The model under review builds one solid part; all positions refer to its coordinate system, in mm. Face numbers are marked on the shaded views. A direction names the side the tool comes from. Give positions to 0.01 mm unless a question says otherwise; leave off trailing zeros. Loops run counter-clockwise (first coordinate to the right, second up) from the corner with the lowest first, then second, coordinate; pieces in that order, holes last. Notation, with made-up numbers: (82.5, 39.25) - (121.5, 39.25) arc R22 cw to (121.5, 45.25) - close; hole circle Ø10 at (88, 36). An arc over 180 degrees is marked (long way). Return JSON: item names as keys, results as strings. Group by question number.
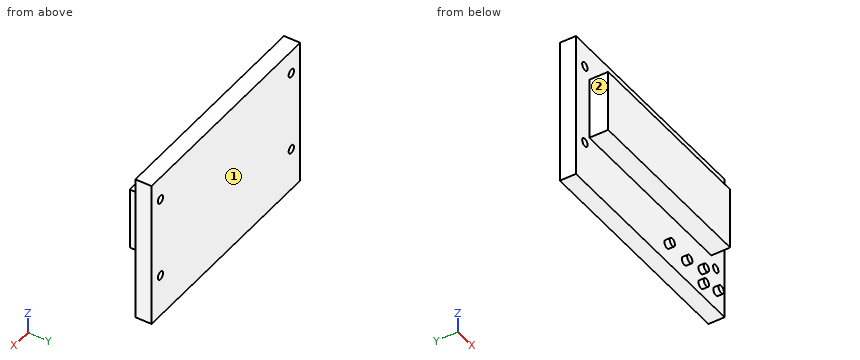
```python
from build123d import *

# Parameters (mm, degrees)
F0_W     = 85.09
F0_H     = 56.134
F0_R     = 1.524
F1_DEPTH = 6.096
F2_W     = 69.85
F2_H     = 23.622
F3_DEPTH = 7.112
F4_R     = 1.5
F5_DEPTH = 2


with BuildPart() as f1:
    # F0 (on Front) → F1 (new body)
    with BuildSketch(Plane.XZ):
        Rectangle(F0_W, F0_H)
        with Locations((-37.465, -11.811)):
            Circle(F0_R, mode=Mode.SUBTRACT)
        with Locations((37.465, -11.811)):
            Circle(F0_R, mode=Mode.SUBTRACT)
        with Locations((-37.465, 19.177)):
            Circle(F0_R, mode=Mode.SUBTRACT)
        with Locations((37.465, 19.177)):
            Circle(F0_R, mode=Mode.SUBTRACT)
    extrude(amount=F1_DEPTH)

    # F2 (on face) → F3 (join)
    with BuildSketch(Plane.XZ.offset(6.096)):
        with Locations((0, 3.683)):
            Rectangle(F2_W, F2_H)
    extrude(amount=F3_DEPTH)

    # F4 (on face) → F5 (join)
    with BuildSketch(Plane.XZ.offset(6.096)):
        with Locations((9.545, -21.067)):
            Circle(F4_R)
        with Locations((19.545, -21.067)):
            Circle(F4_R)
        with Locations((29.045, -24.067)):
            Circle(F4_R)
        with Locations((29.045, -18.067)):
            Circle(F4_R)
        with Locations((37.545, -21.067)):
            Circle(F4_R)
    extrude(amount=F5_DEPTH)


solid = f1.part
```
1) To check wall thickness, follow line 1 (Z direction, x = -38.5, y = -4.25); line 2 (X direction, y = -12, z = 6) (3 decimals); line 3 (Z direction, x = 31.5, y = -8.5). State the ranges of each line that lie inside material, in increasing order.
2) We need section A-A, the plane x = 37. Write out the cut boundary in (y, z).
3) We need section B-B, the plane z = 11. Write out the cut boundary in (x, y) (3 decimals), plus the area to 3 significant figures.
4) For pin 1 Ø1.5 at (x, z) = (29, -19) entering from -Y; pin 2 Ø1.5 at (x, z) = (13.5, -10) entering from +Y; pin 3 Ø3 at (y, z) = (-8, 4.5) entering from +X (3 decimals); pin 4 Ø6 at (x, y) = (16.5, -11) entering from +Z, all flat-tipped, find the tip position at first contact; note any pin that passes through.
5) Tool access review of the marked faces 1 and 2: name each direction out of +Z, -Z, +X, -X, +Y, -Y from which nothing blocks a thin tool from reaching the whole face with its end or side.
6) We need section C-C, the plane y = -7. Write out the cut boundary in (x, z) (3 decimals).
7) We need section D-D, the plane x = -4. Write out the cut boundary in (y, z).
Findings:
{
 "1": {"line 1": "z = -28.07 to -12.93, -10.69 to 18.06, 20.3 to 28.07", "line 2": "x = -34.925 to 34.925", "line 3": "z = -8.13 to 15.49"},
 "2": {"outline": "(-8.1, -22.46) - (-6.1, -22.46) - (-6.1, -28.07) - (0, -28.07) - (0, -13.26) - (-6.1, -13.26) - (-6.1, -19.67) - (-8.1, -19.67) - close; (-6.1, -10.36) - (0, -10.36) - (0, 17.73) - (-6.1, 17.73) - close; (-6.1, 20.63) - (0, 20.63) - (0, 28.07) - (-6.1, 28.07) - close"},
 "3": {"outline": "(-42.545, -6.096) - (-34.925, -6.096) - (-34.925, -13.208) - (34.925, -13.208) - (34.925, -6.096) - (42.545, -6.096) - (42.545, 0) - (-42.545, 0) - close", "area": "1,020 mm^2"},
 "4": {"pin 1": "stops at y = -8.1", "pin 2": "stops at y = 0", "pin 3": "stops at x = 34.925", "pin 4": "stops at z = 15.49"},
 "5": {"face 1": "+Z, -Z, +X, -X, +Y", "face 2": "+Z, -Z, -X, -Y"},
 "6": {"outline": "(-34.925, -8.128) - (34.925, -8.128) - (34.925, 15.494) - (-34.925, 15.494) - close; circle Ø3 at (9.545, -21.067); circle Ø3 at (19.545, -21.067); circle Ø3 at (29.045, -24.067); circle Ø3 at (29.045, -18.067); circle Ø3 at (37.545, -21.067)"},
 "7": {"outline": "(-13.21, -8.13) - (-6.1, -8.13) - (-6.1, -28.07) - (0, -28.07) - (0, 28.07) - (-6.1, 28.07) - (-6.1, 15.49) - (-13.21, 15.49) - close"}
}
